```python
from build123d import *

# Parameters (mm, degrees)
BOSS_EXTRUDE3_DEPTH = 3.175
FILLET1_R           = 3.175


with BuildPart() as part:
    # Sketch1 → Boss-Extrude3 (new body)
    with BuildSketch(Plane.XY):
        with BuildLine():
            Line((35.78531497, 16.139458277), (54.83531497, 16.139458277))
            Line((54.83531497, 16.139458277), (54.83531497, -9.260541723))
            Line((54.83531497, -9.260541723), (-21.36468503, -9.260541723))
            Line((-21.36468503, -9.260541723), (-21.36468503, 16.139458277))
            Line((-21.36468503, 16.139458277), (-2.31468503, 16.139458277))
            ThreePointArc((-2.31468503, 16.139458277), (16.73531497, 35.189458277), (35.78531497, 16.139458277))
        make_face()
    extrude(amount=BOSS_EXTRUDE3_DEPTH)

    # Fillet1
    fillet1_edges = [part.edges().sort_by_distance(p)[0] for p in [
        (54.83531497, 16.139458277, 1.5875),
        (54.83531497, -9.260541723, 1.5875),
        (-21.36468503, -9.260541723, 1.5875),
        (-21.36468503, 16.139458277, 1.5875),
    ]]
    fillet(fillet1_edges, radius=FILLET1_R)


solid = part.part
```
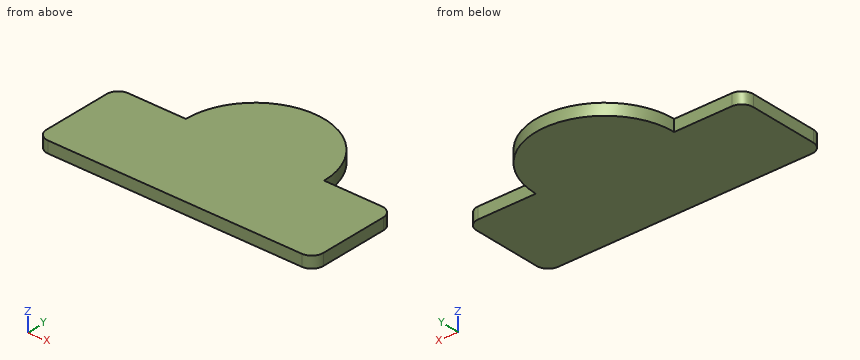
Design review of the part built by this model. Coordinates are the model's own, in mm. Round coordinates to 2 decimals unless told otherwise and drop trailing zeros. Write each loop counter-clockwise with the first axis right and the second up, starting at its lowest first coordinate (ties: lowest second). Pieces come first, ordered by that corner, then holes. Notation, with made-up numbers: (62, -26) -> (112, -26) arc R30 ccw to (112, 3) -> close; hole circle Ø10 at (81, -12.5). An arc over 180 degrees is marked (long way). Answer in a Markdown table with one row per item.
Q1. Take a section at C-C, the plane y = 25.5. State the section outline as (x, z) points (3 decimals).
The answers:
| item | result |
|---|---|
| outline | (0.144, 0) -> (33.327, 0) -> (33.327, 3.175) -> (0.144, 3.175) -> close |
Q2. To check wall thickness, follow L1, parallel to Y at x = -2.5, z = 0.4; L2, parallel to Y at x = 20.5, z = 0.85; L3, parallel to X at y = 27.5, z = 0.45. State the ranges of each line that lie inside material, in increasing order. Write a range as [from, to].
The answers:
| item | result |
|---|---|
| L1 | [-9.26, 16.14] |
| L2 | [-9.26, 34.81] |
| L3 | [1.44, 32.03] |
Q3. Take a section at B-B, the plane x = -9.5. State the section outline as (y, z) points (3 decimals).
The answers:
| item | result |
|---|---|
| outline | (-9.261, 0) -> (16.139, 0) -> (16.139, 3.175) -> (-9.261, 3.175) -> close |
Q4. Clearance check with flat-ended pins moving along their axes: pin 1 Ø4 at (x, y) = (31, 12) entering from -Z; pin 2 Ø1.6 at (x, z) = (41.5, 2.5) entering from +Y. State where each tip first meets the part, or that it passes through.
The answers:
| item | result |
|---|---|
| pin 1 | z = 0 |
| pin 2 | y = 16.14 |
Q5. Take a section at A-A, the plane z = 1.35. State the section outline as (x, y) points (3 decimals), then the cut area to 3 significant figures.
The answers:
| item | result |
|---|---|
| outline | (-21.365, -6.086) arc R3.175 ccw to (-18.19, -9.261) -> (51.66, -9.261) arc R3.175 ccw to (54.835, -6.086) -> (54.835, 12.964) arc R3.175 ccw to (51.66, 16.139) -> (35.785, 16.139) arc R19.05 ccw to (-2.315, 16.139) -> (-18.19, 16.139) arc R3.175 ccw to (-21.365, 12.964) -> close |
| area | 2,500 mm² |
